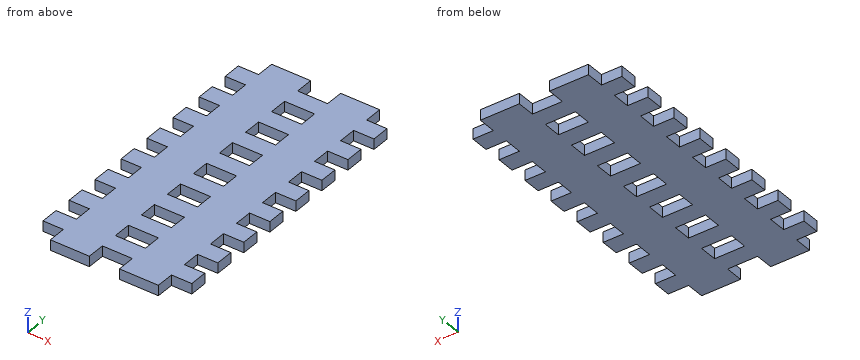
```python
from build123d import *

# Parameters (mm, degrees)
F0_W     = 20.0313134119
F0_H     = 9.17194
F0_H_2   = 9.1719370473
F0_H_3   = 9.1719407726
F0_H_4   = 9.1719385237
F0_H_5   = 9.1719403863
F0_H_6   = 9.1719399947
F0_H_7   = 9.1719411589
F0_H_8   = 9.1719400741
F0_W_2   = 20.0313036
F0_W_3   = 15.4139306396
F0_W_4   = 10.4550179094
F0_W_5   = 10.4550202707
F0_W_6   = 10.455021
F1_DEPTH = 5.334


# Not quite as in the source:
# - ends of sketch curves that miss each other by under 0.0002 mm in the source are joined


with BuildPart() as f1:
    # F0 (on Top) → F1 (new body)
    with BuildSketch(Plane.XY):
        with Locations((-17.7226220258, 74.8951544916)):
            Rectangle(F0_W, F0_H)
        with Locations((-17.7226220258, 65.723215968)):
            Rectangle(F0_W, F0_H_2)
        with Locations((-17.7226220258, 47.3793366717)):
            Rectangle(F0_W, F0_H)
        with Locations((-17.7226220258, 56.551277058)):
            Rectangle(F0_W, F0_H_3)
        with Locations((-17.7226220258, 38.2073974099)):
            Rectangle(F0_W, F0_H_4)
        with Locations((-17.7226220258, 29.0354579549)):
            Rectangle(F0_W, F0_H_5)
        with Locations((-17.7226220258, -16.824242307)):
            Rectangle(F0_W, F0_H)
        with Locations((-17.7226220258, 1.5196376903)):
            Rectangle(F0_W, F0_H_6)
        with Locations((-17.7226220258, -35.1681232728)):
            Rectangle(F0_W, F0_H_7)
        with Locations((-17.7226220258, 10.6915776877)):
            Rectangle(F0_W, F0_H)
        with Locations((-17.7226220258, -7.652302307)):
            Rectangle(F0_W, F0_H)
        with Locations((-17.7226220258, -53.5120038522)):
            Rectangle(F0_W, F0_H)
        with Locations((-17.7226220258, -25.9961825002)):
            Rectangle(F0_W, F0_H_5)
        with Locations((-17.7226220258, -44.3400638522)):
            Rectangle(F0_W, F0_H)
        with Locations((-17.7226220258, -62.6839438522)):
            Rectangle(F0_W, F0_H)
        with Locations((-17.7226220258, 19.8635177247)):
            Rectangle(F0_W, F0_H_8)
        with Locations((17.7226171198, 29.0354579549)):
            Rectangle(F0_W_2, F0_H_5)
        with Locations((17.7226171198, 47.3793366717)):
            Rectangle(F0_W_2, F0_H)
        with Locations((17.7226171198, -62.6839438522)):
            Rectangle(F0_W_2, F0_H)
        with Locations((17.7226171198, 19.8635177247)):
            Rectangle(F0_W_2, F0_H_8)
        with Locations((17.7226171198, -53.5120038522)):
            Rectangle(F0_W_2, F0_H)
        with Locations((17.7226171198, -25.9961825002)):
            Rectangle(F0_W_2, F0_H_5)
        with Locations((17.7226171198, -7.652302307)):
            Rectangle(F0_W_2, F0_H)
        with Locations((17.7226171198, 38.2073974099)):
            Rectangle(F0_W_2, F0_H_4)
        with Locations((17.7226171198, -35.1681232728)):
            Rectangle(F0_W_2, F0_H_7)
        with Locations((17.7226171198, 10.6915776877)):
            Rectangle(F0_W_2, F0_H)
        with Locations((17.7226171198, -44.3400638522)):
            Rectangle(F0_W_2, F0_H)
        with Locations((17.7226171198, 65.723215968)):
            Rectangle(F0_W_2, F0_H_2)
        with Locations((17.7226171198, 74.8951544916)):
            Rectangle(F0_W_2, F0_H)
        with Locations((17.7226171198, 56.551277058)):
            Rectangle(F0_W_2, F0_H_3)
        with Locations((17.7226171198, -16.824242307)):
            Rectangle(F0_W_2, F0_H)
        with Locations((17.7226171198, 1.5196376903)):
            Rectangle(F0_W_2, F0_H_6)
        Polygon((27.7382689198, 70.3091844916), (27.7382689198, 61.1372474443), (38.1932891905, 61.1372474443), (38.1932891905, 70.3091878306), align=None)
        with Locations((0, 65.723215968)):
            Rectangle(F0_W_3, F0_H_2)
        with Locations((-32.9657876864, 65.723215968)):
            Rectangle(F0_W_4, F0_H_2)
        with Locations((-32.9657876864, 47.3793366717)):
            Rectangle(F0_W_4, F0_H)
        with Locations((0, 47.3793366717)):
            Rectangle(F0_W_3, F0_H)
        with Locations((32.9657790552, 47.3793366717)):
            Rectangle(F0_W_5, F0_H)
        with Locations((32.9657790552, 29.0354579549)):
            Rectangle(F0_W_5, F0_H_5)
        with Locations((0, 29.0354579549)):
            Rectangle(F0_W_3, F0_H_5)
        with Locations((-32.9657876864, 29.0354579549)):
            Rectangle(F0_W_4, F0_H_5)
        with Locations((-32.9657876864, 10.6915776877)):
            Rectangle(F0_W_4, F0_H)
        with Locations((32.9657790552, 10.6915776877)):
            Rectangle(F0_W_5, F0_H)
        with Locations((32.9657790552, -7.652302307)):
            Rectangle(F0_W_5, F0_H)
        with Locations((-32.9657876864, -7.652302307)):
            Rectangle(F0_W_4, F0_H)
        with Locations((-32.9657876864, -25.9961825002)):
            Rectangle(F0_W_4, F0_H_5)
        with Locations((0, 10.6915776877)):
            Rectangle(F0_W_3, F0_H)
        with Locations((0, -7.652302307)):
            Rectangle(F0_W_3, F0_H)
        with Locations((0, -25.9961825002)):
            Rectangle(F0_W_3, F0_H_5)
        with Locations((0, -44.3400638522)):
            Rectangle(F0_W_3, F0_H)
        with Locations((32.9657794198, -25.9961825002)):
            Rectangle(F0_W_6, F0_H_5)
        with Locations((32.9657794198, -44.3400638522)):
            Rectangle(F0_W_6, F0_H)
        with Locations((-32.9657876864, -44.3400638522)):
            Rectangle(F0_W_4, F0_H)
        with Locations((-32.9657876864, -62.6839438522)):
            Rectangle(F0_W_4, F0_H)
        with Locations((0, -62.6839438522)):
            Rectangle(F0_W_3, F0_H)
        with Locations((32.9657794198, -62.6839438522)):
            Rectangle(F0_W_6, F0_H)
        with Locations((-17.7226220258, -71.8558840454)):
            Rectangle(F0_W, F0_H_5)
        with Locations((17.7226171198, -71.8558840454)):
            Rectangle(F0_W_2, F0_H_5)
    extrude(amount=F1_DEPTH)


solid = f1.part
```
Part model, mm, in its own coordinate system. Give positions to 0.01 mm unless a question says otherwise; leave off trailing zeros. Write each loop counter-clockwise with the first axis right and the second up, starting at its lowest first coordinate (ties: lowest second). Pieces come first, ordered by that corner, then holes. Notation, with made-up numbers: (24, 78.25) -> (51, 78.25) arc R17 cw to (51, 99.25) -> close; hole circle Ø5 at (49.5, 66.5). An arc over 180 degrees is marked (long way). Put each result on its own line as item: value. Start each with the question number.
Item 1: Cut at A-A (x = 32). State how many separate pieces and enclosed holes the cut face has, then the cut area to 3 significant figures.
Item 2: Cut at B-B (y = -19). List the corners of the cut face in (x, z).
Item 3: Wall check: L1, parallel to X at y = 59, z = 3.7. Give the ranges that are in metal, low to high. Write a range as [from, to].
Item 4: Pin check, flat tips, straight feed: pin 1 Ø2.5 at (x, z) = (0.5, 3.5) entering from -Y; pin 2 Ø1.6 at (y, z) = (56, 2) entering from -X; pin 3 Ø2.5 at (x, z) = (-2, 2) entering from +Y. Stop position of each tip, or through.
Answer list:
1. separate pieces: 8
1. enclosed holes: 0
1. area: 391 mm2
2. outline: (-27.74, 0) -> (-7.71, 0) -> (-7.71, 5.33) -> (-27.74, 5.33) -> close; (7.71, 0) -> (27.74, 0) -> (27.74, 5.33) -> (7.71, 5.33) -> close
3. L1: x = [-27.74, -7.71], [7.71, 27.74]
4. pin 1: stops at y = -67.27
4. pin 2: stops at x = -27.74
4. pin 3: stops at y = 70.31
